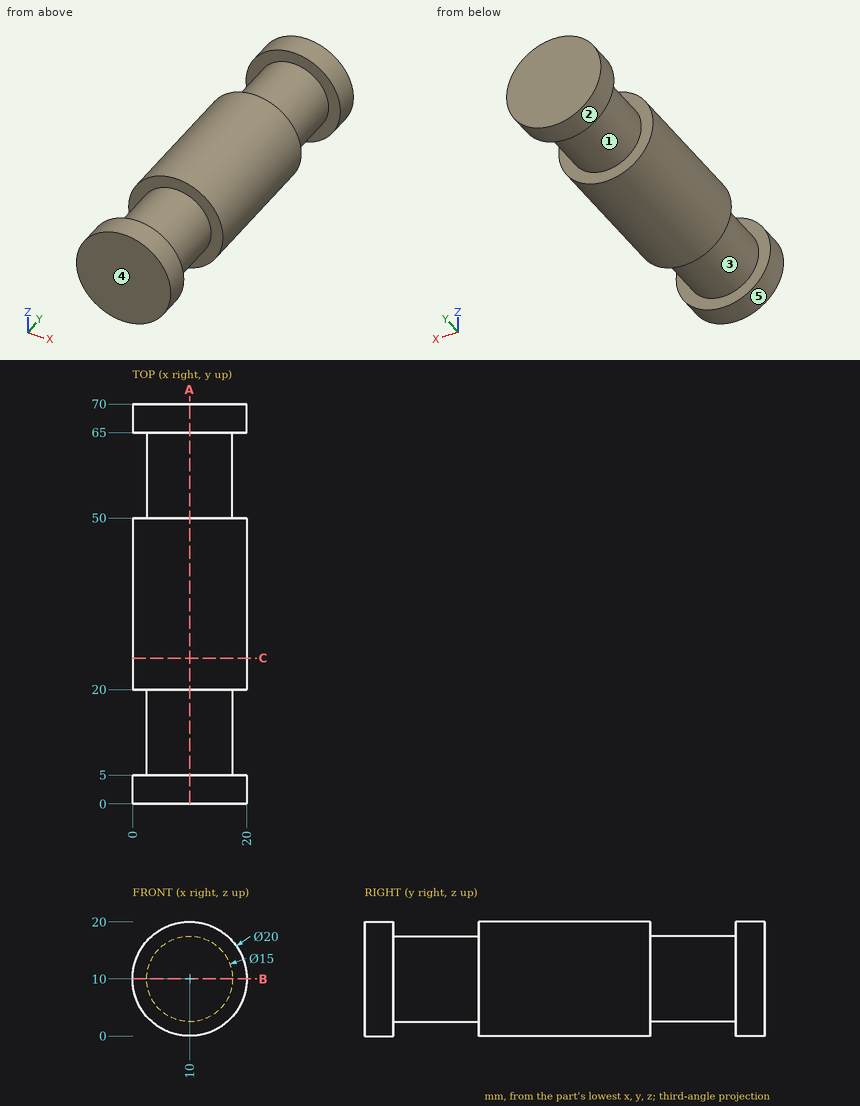
For this review, use the dimensioned drawing (mm, ordinates from the lowest corner) and the shaded views. A direction names the side the tool comes from. Give positions to 0.01 mm unless a question says otherwise; leave off trailing zeros. Order: outer loops, then holes, each group sorted by start corner. A loop starts at its lowest first (then second) coordinate and runs counter-clockwise, first axis right, second up. Notation, with made-up numbers: M 43.25,53.5 L 83.25,53.5 A26 ccw 83.25,83.5 Z; hole C -12,64.25 d6. An arc over 180 degrees is marked long. One line per question, with ' | ' between items. Start each with the question number.
1) Mouldability with a two-part tool opening along Y and no side actions: class the marked faces 3, 4 and 5 as pulls with the +Y half, pulls with the -Y half, needs draft (parallel to the pull), parting line crosses it, or undercut.
2) Wall thickness on L1, parallel to Y at x = 3.25, z = 6.25; L2, parallel to Z at x = 10.5, y = 46.5; L3, parallel to Z at x = 10.25, y = 53: over which ranges is each line inside the solid? List them lowest first. Write a range as from..to.
3) Consider section A-A, the plane x = 10. Give the boundary of the cut face in (y, z), then the cut area to 3 significant figures.
4) Consider section B-B, the plane z = 10. Give the boundary of the cut face in (x, y).
5) For the marked faces 1 and 2, list the 3-axis set-ups (+Z, -Z, +X, -X, +Y, -Y) from which the entire face can be reached by the end or side of a thin tool; tool diameter is ignored.
6) Clearance check with flat-ended pins moving along their axes: P1, Ø12, axis at x = 14, z = 4, coming from the -Y side; P2, Ø1, axis at x = 3, y = 24, coming from the -Z side; P3, Ø5, axis at x = 14.5, y = 9, coming from the -Z side; P4, Ø10, axis at x = 14, y = 15.5, coming from the -Z side. State where each tip first meets the part, or that it passes through.
7) Consider section C-C, the plane y = 25.5. Give the boundary of the cut face in (x, z), then the cut area to 3 significant figures.
Found:
1) face 3: undercut | face 4: pulls with the -Y half | face 5: needs draft
2) L1: y = 0..5, 20..50, 65..70 | L2: z = 0.01..19.99 | L3: z = 2.5..17.5
3) outline: M 0,0 L 5,0 L 5,2.5 L 20,2.5 L 20,0 L 50,0 L 50,2.5 L 65,2.5 L 65,0 L 70,0 L 70,20 L 65,20 L 65,17.5 L 50,17.5 L 50,20 L 20,20 L 20,17.5 L 5,17.5 L 5,20 L 0,20 Z | area: 1,250 mm²
4) outline: M 0,0 L 20,0 L 20,5 L 17.5,5 L 17.5,20 L 20,20 L 20,50 L 17.5,50 L 17.5,65 L 20,65 L 20,70 L 0,70 L 0,65 L 2.5,65 L 2.5,50 L 0,50 L 0,20 L 2.5,20 L 2.5,5 L 0,5 Z
5) face 1: none | face 2: +Y, -Y
6) P1: stops at y = 0 | P2: stops at z = 2.4 | P3: stops at z = 2.77 | P4: stops at z = 0.17
7) outline: C 10,10 d20 | area: 314 mm²
